```python
from build123d import *

# Parameters (mm, degrees)
BOSS_EXTRUDE1_DEPTH = 30
CUT_EXTRUDE1_DEPTH  = 3.8
CUT_EXTRUDE2_DEPTH  = 3.8
CUT_EXTRUDE3_DEPTH  = 3.8
CUT_EXTRUDE4_DEPTH  = 3.8
SKETCH11_R          = 4.5
CUT_EXTRUDE5_DEPTH  = 2.1
SKETCH12_R          = 4.5
CUT_EXTRUDE6_DEPTH  = 2.1
SKETCH15_R          = 4.8
BOSS_EXTRUDE2_DEPTH = 2
CUT_EXTRUDE7_DEPTH  = 3


with BuildPart() as part:
    # Sketch1 → Boss-Extrude1 (new body)
    with BuildSketch(Plane.XY):
        with BuildLine():
            Line((0, 0), (120, 0))
            Line((120, 0), (120, 88.5))
            Line((120, 88.5), (26.3, 88.5))
            ThreePointArc((26.3, 88.5), (12.762673874, 86.869132207), (0, 82.069852679))
            Line((0, 82.069852679), (0, 0))
        make_face()
    extrude(amount=-BOSS_EXTRUDE1_DEPTH)

    # Sketch2 → Cut-Revolve1 (revolve, cut)
    with BuildSketch(Plane(origin=(42, 0, 0), x_dir=(0, 0, -1), z_dir=(1, 0, 0))):
        Polygon((0, 41.5), (0, 57.366025404), (1.5, 56.5), (23, 56.5), (23, 41.5), align=None)
    revolve(axis=Axis((42, 41.5, -23), (0, 0, 1)), mode=Mode.SUBTRACT)

    # Sketch3 → Cut-Revolve2 (revolve, cut)
    with BuildSketch(Plane(origin=(100.5, 0, 0), x_dir=(0, 0, -1), z_dir=(1, 0, 0))):
        Polygon((26.2, 8), (29.2, 11), (29.2, 12.4), (28.6, 13), (23.2, 13), (23.2, 13.5), (30, 13.5), (30, 8), align=None)
    revolve(axis=Axis((100.5, 8, -30), (0, 0, 1)), mode=Mode.SUBTRACT)

    # Sketch4 → Cut-Revolve3 (revolve, cut)
    with BuildSketch(Plane(origin=(16.5, 0, 0), x_dir=(0, 0, -1), z_dir=(1, 0, 0))):
        Polygon((26.2, 6.5), (29.2, 9.5), (29.2, 10.9), (28.6, 11.5), (23.2, 11.5), (23.2, 12), (30, 12), (30, 6.5), align=None)
    revolve(axis=Axis((16.5, 6.5, -30), (0, 0, 1)), mode=Mode.SUBTRACT)

    # Sketch5 → Cut-Revolve4 (revolve, cut)
    with BuildSketch(Plane(origin=(108.5, 0, 0), x_dir=(0, 0, -1), z_dir=(1, 0, 0))):
        Polygon((26.2, 58), (29.2, 61), (29.2, 62.4), (28.6, 63), (23.2, 63), (23.2, 63.5), (30, 63.5), (30, 58), align=None)
    revolve(axis=Axis((108.5, 58, -30), (0, 0, 1)), mode=Mode.SUBTRACT)

    # Sketch6 → Cut-Revolve5 (revolve, cut)
    with BuildSketch(Plane(origin=(13, 0, 0), x_dir=(0, 0, -1), z_dir=(1, 0, 0))):
        Polygon((26.2, 49), (29.2, 52), (29.2, 53.4), (28.6, 54), (23.2, 54), (23.2, 54.5), (30, 54.5), (30, 49), align=None)
    revolve(axis=Axis((13, 49, -30), (0, 0, 1)), mode=Mode.SUBTRACT)

    # Sketch7 → Cut-Extrude1 (cut)
    with BuildSketch(Plane.XY.offset(-30)):
        Polygon((98, 9.443375673), (98, 6.556624327), (100.5, 5.113248654), (103, 6.556624327), (103, 9.443375673), (100.5, 10.886751346), align=None)
    extrude(amount=CUT_EXTRUDE1_DEPTH, mode=Mode.SUBTRACT)

    # Sketch8 → Cut-Extrude2 (cut)
    with BuildSketch(Plane.XY.offset(-30)):
        Polygon((14, 7.943375673), (14, 5.056624327), (16.5, 3.613248654), (19, 5.056624327), (19, 7.943375673), (16.5, 9.386751346), align=None)
    extrude(amount=CUT_EXTRUDE2_DEPTH, mode=Mode.SUBTRACT)

    # Sketch9 → Cut-Extrude3 (cut)
    with BuildSketch(Plane.XY.offset(-30)):
        Polygon((106, 59.443375673), (106, 56.556624327), (108.5, 55.113248654), (111, 56.556624327), (111, 59.443375673), (108.5, 60.886751346), align=None)
    extrude(amount=CUT_EXTRUDE3_DEPTH, mode=Mode.SUBTRACT)

    # Sketch10 → Cut-Extrude4 (cut)
    with BuildSketch(Plane.XY.offset(-30)):
        Polygon((10.5, 50.443375673), (10.5, 47.556624327), (13, 46.113248654), (15.5, 47.556624327), (15.5, 50.443375673), (13, 51.886751346), align=None)
    extrude(amount=CUT_EXTRUDE4_DEPTH, mode=Mode.SUBTRACT)

    # Sketch11 → Cut-Extrude5 (cut)
    with BuildSketch(Plane.XY.offset(-30)):
        with Locations((80, 21)):
            Circle(SKETCH11_R)
    extrude(amount=CUT_EXTRUDE5_DEPTH, mode=Mode.SUBTRACT)

    # Sketch12 → Cut-Extrude6 (cut)
    with BuildSketch(Plane.XY.offset(-30)):
        with Locations((40, 21)):
            Circle(SKETCH12_R)
    extrude(amount=CUT_EXTRUDE6_DEPTH, mode=Mode.SUBTRACT)

    # Sketch13 → Cut-Revolve6 (revolve, cut)
    with BuildSketch(Plane(origin=(0, 21, 0), x_dir=(1, 0, 0), z_dir=(0, 1, 0))):
        Polygon((100, 30), (104, 30), (103.3235, 29.3235), (103.3235, 8), (100, 6.08117638), align=None)
    revolve(axis=Axis((100, 21, -6.08117638), (0, 0, -1)), mode=Mode.SUBTRACT)

    # Sketch14 → Cut-Revolve7 (revolve, cut)
    with BuildSketch(Plane(origin=(0, 21, 0), x_dir=(1, 0, 0), z_dir=(0, 1, 0))):
        Polygon((20, 30), (24, 30), (23.3235, 29.3235), (23.3235, 8), (20, 6.08117638), align=None)
    revolve(axis=Axis((20, 21, -6.08117638), (0, 0, -1)), mode=Mode.SUBTRACT)

    # Sketch15 → Boss-Extrude2 (add)
    with BuildSketch(Plane.XY):
        with Locations((23, 81.5)):
            Circle(SKETCH15_R)
    extrude(amount=BOSS_EXTRUDE2_DEPTH)

    # Sketch16 → Cut-Revolve8 (revolve, cut)
    with BuildSketch(Plane(origin=(54.5, 0, 0), x_dir=(0, 0, -1), z_dir=(1, 0, 0))):
        Polygon((5, 88.5), (2.806572993, 88.5), (2.612213504, 88.387786496), (2.5, 88.5), (2.5, 89.5), (5, 89.5), align=None)
    revolve(axis=Axis((54.5, 89.5, -5), (0, -1, 0)), mode=Mode.SUBTRACT)

    # Sketch17 → Cut-Extrude7 (cut)
    with BuildSketch(Plane(origin=(0, 88.5, 0), x_dir=(1, 0, 0), z_dir=(0, 1, 0))):
        Polygon((53.25, 5.721687836), (53.25, 4.278312164), (54.5, 3.556624327), (55.75, 4.278312164), (55.75, 5.721687836), (54.5, 6.443375673), align=None)
    extrude(amount=-CUT_EXTRUDE7_DEPTH, mode=Mode.SUBTRACT)


solid = part.part
```
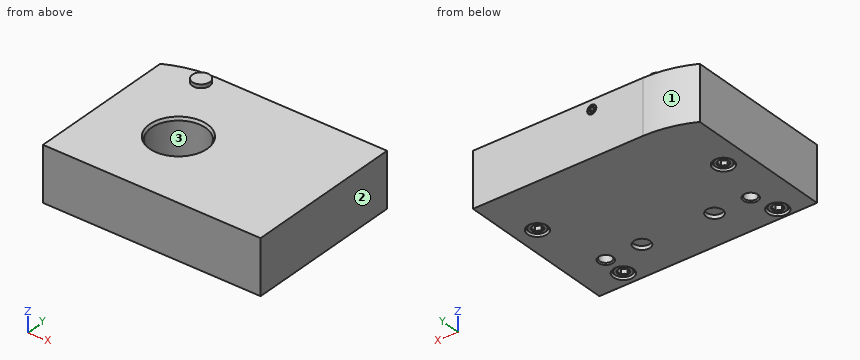
Part model, mm, in its own coordinate system. Face numbers are marked on the shaded views. Round coordinates to 2 decimals unless told otherwise and drop trailing zeros. Order: outer loops, then holes, each group sorted by start corner. A loop starts at its lowest first (then second) coordinate and runs counter-clockwise, first axis right, second up. Notation, with made-up numbers: M 26,32 L 71,32 A14 cw 71,41 Z; hole C -19,44.25 d8. An arc over 180 degrees is marked long. Put each result on its own line as item: value. Start each with the question number.
1. Drop flat-ended pins along their axis: pin 1 (2.5 mm diameter, centred on x = 109, y = 58.5, fed in from -Z); pin 2 (7.5 mm diameter, centred on x = 100, y = 21, fed in from +Z); pin 3 (4.5 mm diameter, centred on x = 80.5, y = 23, fed in from -Z); pin 4 (14.5 mm diameter, centred on x = 40, y = 21, fed in from -Z). Give the stop position or say it passes through.
2. Two-plate mould, pull along Y, no slides. Class the marked faces 1, 2 and 3: +Y half, -Y half, draft (parallel to the pull), parting line (faces both ways), or undercut.
3. Slice it at A-A on z = -10. List the corners of the cut face in (x, y).
4. Slice it at C-C on x = 80. List the corners of the cut face in (y, z), then the cut area to 3 significant figures.
5. Slice it at B-B on x = 42. List the corners of the cut face in (y, z).
6. Drill centre lines: probe 1 along X at (y, z) = (49, -27.75); probe 2 along Y at (x, z) = (40, -28.35); probe 3 along Y at (x, z) = (109.5, -26). Where is each one in solid material? Low to high. Write a range as [from, to].
Findings:
1. pin 1: z = -26.2
1. pin 2: z = 0
1. pin 3: z = -27.9
1. pin 4: z = -30
2. face 1: +Y half
2. face 2: draft
2. face 3: undercut
3. outline: M 0,0 L 120,0 L 120,88.5 L 26.3,88.5 A57 ccw 0,82.07 Z; hole C 20,21 d6.65; hole C 42,41.5 d30; hole C 100,21 d6.65
4. outline: M 0,-30 L 16.5,-30 L 16.5,-27.9 L 25.5,-27.9 L 25.5,-30 L 88.5,-30 L 88.5,0 L 0,0 Z
4. area: 2,640 mm2
5. outline: M 0,-30 L 16.97,-30 L 16.97,-27.9 L 25.03,-27.9 L 25.03,-30 L 88.5,-30 L 88.5,0 L 57.37,0 L 56.5,-1.5 L 56.5,-23 L 26.5,-23 L 26.5,-1.5 L 25.63,0 L 0,0 Z
6. probe 1: [0, 7.5], [8, 10.5], [15.5, 18], [18.5, 120]
6. probe 2: [0, 16.5], [25.5, 88.5]
6. probe 3: [0, 52.59], [53.1, 62.9], [63.41, 88.5]
